CAD build for the part. Positions are in the model's coordinates, mm. Give positions to 0.01 mm unless a question says otherwise; leave off trailing zeros. Write each loop counter-clockwise with the first axis right and the second up, starting at its lowest first coordinate (ties: lowest second). Pieces come first, ordered by that corner, then holes. Notation, with made-up numbers: (-19, 50.5) -> (28, 50.5) arc R12 ccw to (28, 71.5) -> close; hole circle Ø3 at (83.25, 65). An arc over 180 degrees is marked (long way). Answer as a JSON object with one key per item and string values.
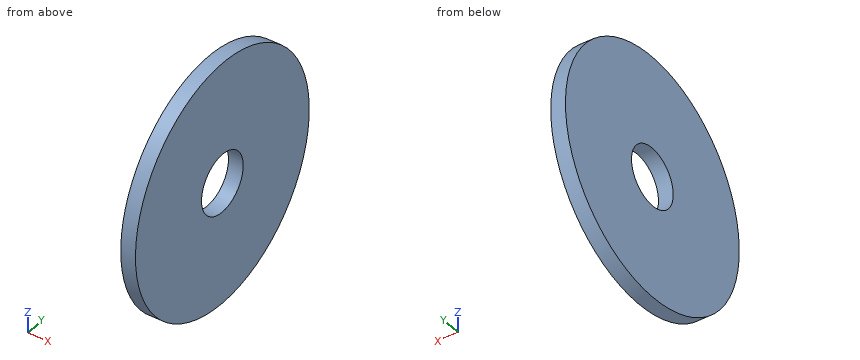
```python
from build123d import *

# Parameters (mm, degrees)
CYLINDER007_R           = 6
CYLINDER007_DEPTH       = 236
CYLINDER007_PITCH_ANGLE = 90
CYLINDER002_R           = 25
CYLINDER002_DEPTH       = 3
CYLINDER002_PITCH_ANGLE = 90


with BuildPart() as connector_bore:
    # Cylinder007 → Cylinder007 (new body)
    with BuildSketch(Plane.XY):
        Circle(CYLINDER007_R)
    extrude(amount=CYLINDER007_DEPTH)


with BuildPart() as connector_bore_1:
    # Cylinder007 pitch: moved
    add(connector_bore.part.rotate(Axis((0, 0, 0), (0, 1, 0)), CYLINDER007_PITCH_ANGLE))


with BuildPart() as connector_bore_2:
    # Cylinder007 placement: moved
    add(connector_bore_1.part.moved(Location((-45, 0, 0))))


with BuildPart() as cut005:
    # Cylinder002 → Cylinder002 (new body)
    with BuildSketch(Plane.XY):
        Circle(CYLINDER002_R)
    extrude(amount=CYLINDER002_DEPTH)


with BuildPart() as cut005_1:
    # Cylinder002 pitch: moved
    add(cut005.part.rotate(Axis((0, 0, 0), (0, 1, 0)), CYLINDER002_PITCH_ANGLE))


with BuildPart() as cut005_2:
    # Cylinder002 placement: moved
    add(cut005_1.part.moved(Location((150, 0, 0))))

    # Cut005: cut connector_bore
    add(connector_bore_2.part, mode=Mode.SUBTRACT)


solid = cut005_2.part
```
1) Slice it at D-D (y = -15). List the corners of the cut face in (x, z).
Model answer:
{"outline": "(150, -20) -> (153, -20) -> (153, 20) -> (150, 20) -> close"}
2) Wall check: probe 1 along Y at (x, z) = (151.9, 0); probe 2 along Z at (x, y) = (150.45, -1.5); probe 3 along Z at (x, y) = (150.9, 3). Give the ranges that are in metal, low to high.
Model answer:
{"probe 1": "y = -25 to -6, 6 to 25", "probe 2": "z = -24.95 to -5.81, 5.81 to 24.95", "probe 3": "z = -24.82 to -5.2, 5.2 to 24.82"}
3) Pin check, flat tips, straight feed: pin 1 (1.5 mm diameter, centred on x = 151.5, y = 5, fed in from +Z); pin 2 (1 mm diameter, centred on x = 150.5, z = -7, fed in from -Y); pin 3 (1 mm diameter, centred on x = 151.5, z = 10, fed in from +Y). Stop position of each tip, or through.
Model answer:
{"pin 1": "stops at z = 24.64", "pin 2": "stops at y = -24.14", "pin 3": "stops at y = 23.12"}
4) Slice it at C-C (x = 151.8). List the corners of the cut face in (y, z).
Model answer:
{"outline": "circle Ø50 at (0, 0); hole circle Ø12 at (0, 0)"}
5) Slice it at A-A (z = 0). List the corners of the cut face in (x, y), then the cut area to 3 significant figures.
Model answer:
{"outline": "(150, -25) -> (153, -25) -> (153, -6) -> (150, -6) -> close; (150, 6) -> (153, 6) -> (153, 25) -> (150, 25) -> close", "area": "114 mm2"}
